```python
from build123d import *

# Parameters (mm, degrees)
F0_R     = 51.5
F0_R_2   = 50
F1_DEPTH = 45
F2_DEPTH = 200
F3_DEPTH = 5
F4_T     = 2.5


# Not quite as in the source:
# - a shell that OpenCascade refuses in one call is made with other operations: the cavity is built on its own and cut out


with BuildPart() as f1:
    # F0 (on Right) → F1 (new body)
    with BuildSketch(Plane.YZ):
        Circle(F0_R)
        Circle(F0_R_2, mode=Mode.SUBTRACT)
    extrude(amount=F1_DEPTH)

    # F0 (on Right) → F2 (join)
    with BuildSketch(Plane.YZ):
        Circle(F0_R_2)
    extrude(amount=F2_DEPTH)

    # F0 (on Right) → F3 (join)
    with BuildSketch(Plane.YZ):
        Circle(F0_R)
        Circle(F0_R_2, mode=Mode.SUBTRACT)
    extrude(amount=-F3_DEPTH)

    # F4: shell of thickness 2.5, made by hand


with BuildPart() as f4_core1:
    # F4_t2: copy of F1
    add(f1.part)

    # the walls: a layer under each face that stays
    f4_faces = [f4_core1.faces().sort_by_distance(p)[0] for p in [
        (22.5, -51.5, 0),
        (-2.5, -51.5, 0),
        (45, 45.0625, -24.7962962963),
        (-5, 45.0625, -24.7962962963),
        (122.5, -50, 0),
        (-2.5, -50, 0),
        (200, 0, 0),
    ]]
    thicken(f4_faces, amount=-F4_T, mode=Mode.SUBTRACT)

    # F4_s3 → F4_t4 (revolve, cut)
    with BuildSketch(Plane.XY):
        Polygon((45.025, 50.025), (42.5, 50), (42.5, 47.5), (45, 47.5), align=None)
    revolve(axis=Axis((45, 0, 0), (1, 0, 0)), mode=Mode.SUBTRACT)


with BuildPart() as f1_1:
    add(f1.part)

    # what is left inside the walls is the cavity
    f4_cavity = [f4_core1.part.solids().sort_by_distance(p)[0] for p in [
        (146.666667, -47.475, 0),
    ]]
    add(f4_cavity, mode=Mode.SUBTRACT)


solid = f1_1.part
```
Here's how the part is built. I have some questions about the finished solid (model axes, mm). A direction names the side the tool comes from. Coordinates: 2 decimals unless noted, no trailing zeros. Loops run counter-clockwise (first coordinate to the right, second up) from the corner with the lowest first, then second, coordinate; pieces in that order, holes last. Notation, with made-up numbers: (7, 83) - (11, 83) arc R33 cw to (11, 115) - close; hole circle Ø11 at (-33, -19.75). An arc over 180 degrees is marked (long way). Return JSON: item names as keys, results as strings. Group by question number.
Item 1: On a 3-axis mill with a long thin cutter (end or side, diameter ignored), from which of +Z, -Z, +X, -X, +Y, -Y can I reach the whole of each face in a straight line? I mean faces 4 (the face through (45, -8, 50)), 5 (the face through (0, 37, -33)), 6 (the face through (20.35, -11.164, -50.275)). Say none if no direction works.
Item 2: I need wall thicknesses on line 1 (Z direction, x = -2.55, y = 0); line 2 (Z direction, x = 17, y = 0); line 3 (X direction, y = -19.5, z = 43). Which ranges of each line are inside material? Lowest first, please. Write a range as from..to.
Item 3: If we section it at A-A on y = 0: Write out the boundary of the cut face in (x, z).
Item 4: We'd pull the mould along Y, two halves only. Please class faces 1 (the face through (121.42, 47.69, 15.02)), 2 (the face through (-5, -8, 50)), 3 (the face through (-2.46, 47.69, 15.02)): +Y half, -Y half, draft (parallel to the pull), parting line (faces both ways), or undercut.
Item 5: If we section it at C-C on x = 95: Write out the boundary of the cut face in (y, z).
Item 6: Will these pins go through, and if not, where does the flat tip stop? P1, Ø10, axis at x = 121.5, z = 37, coming from the +Y side; P2, Ø5, axis at x = 139.5, z = 28.5, coming from the +Y side; P3, Ø8, axis at x = 164, y = 9.5, coming from the +Z side.
Calculated:
{
 "1": {"face 4": "+X", "face 5": "-X", "face 6": "+X, -X"},
 "2": {"line 1": "z = -51.5..-50, 50..51.5", "line 2": "z = -51.5..-49, 49..51.5", "line 3": "x = 197.5..200"},
 "3": {"outline": "(-5, -51.5) - (45, -51.5) - (45, -50) - (200, -50) - (200, 50) - (45, 50) - (45, 51.5) - (-5, 51.5) - (-5, 50) - (0, 50) - (0, 49) - (42.5, 49) - (42.5, 47.5) - (197.5, 47.5) - (197.5, -47.5) - (42.5, -47.5) - (42.5, -49) - (0, -49) - (0, -50) - (-5, -50) - close"},
 "4": {"face 1": "parting line", "face 2": "draft", "face 3": "undercut"},
 "5": {"outline": "circle Ø100 at (0, 0); hole circle Ø95 at (0, 0)"},
 "6": {"P1": "stops at y = 38.42", "P2": "stops at y = 42.71", "P3": "stops at z = 49.7"}
}
